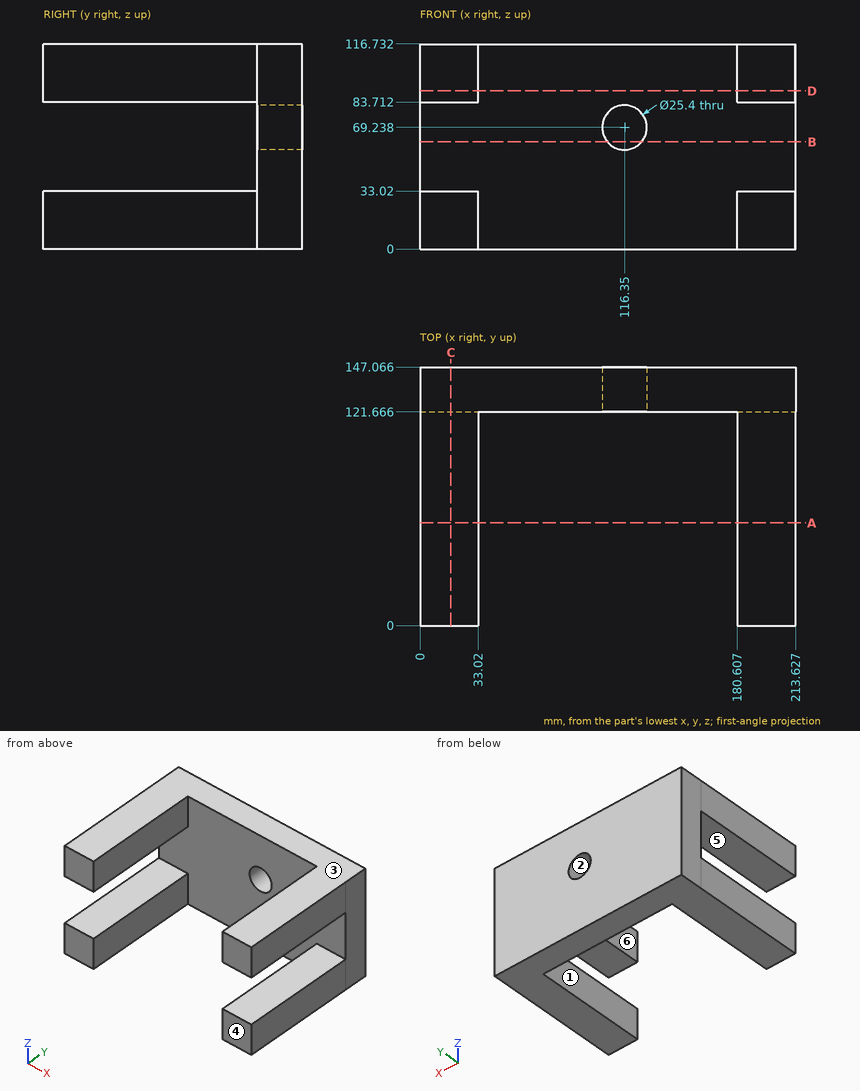
Can you work these out from the drawing? Everything is in mm from the part's minimum corner. A direction names the side the tool comes from. Round coordinates to 2 decimals unless told otherwise and drop trailing zeros. Order: outer loops, then holes, each group sorted by start corner. A loop starts at its lowest first (then second) coordinate and runs counter-clockwise, first axis right, second up. Notation, with made-up numbers: (63, 6.5) -> (114, 6.5) arc R26 ccw to (114, 40.5) -> close; hole circle Ø10 at (-36, 68). An arc over 180 degrees is marked (long way). Return JSON: item names as keys, results as strings. Group by question number.
1. I need wall thicknesses on line 1 (X direction, y = 59, z = 10.5); line 2 (Z direction, x = 205, y = 98); line 3 (Y direction, x = 205.5, z = 36). Which ranges of each line are inside material? Lowest first, please. Write a range as [from, to].
2. We'd pull the mould along Z, two halves only. Please class the marked faces 1, 2 and 3: released by +Z, released by -Z, zero draft, split by the parting line, or undercut.
3. If we section it at A-A, the plane y = 58.5: Write out the boundary of the cut face in (x, z), then the cut area to 3 significant figures.
4. If we section it at D-D, the plane z = 90: Write out the boundary of the cut face in (x, y), then the cut area to 3 significant figures.
5. Will this pin go through, and if not, where does the flat tip stop? pin 1 (6 mm diameter, centred on x = 35.5, z = 11.5, fed in from -Y).
6. If we section it at C-C, the plane x = 17.5: Write out the boundary of the cut face in (y, z), then the cut area to 3 significant figures.
7. If we section it at B-B, the plane z = 61: Write out the boundary of the cut face in (x, y) (1 decimal).
8. Which directions (+Z, -Z, +X, -X, +Y, -Y) give clear straight access to the entire face, cutting with the end or side of a thin tool? Please do the marked faces 4, 5 and 6.
Output values:
{
 "1": {"line 1": "[0, 33.02], [180.61, 213.63]", "line 2": "[0, 33.02], [83.71, 116.73]", "line 3": "[121.67, 147.07]"},
 "2": {"face 1": "zero draft", "face 2": "undercut", "face 3": "released by +Z"},
 "3": {"outline": "(0, 0) -> (33.02, 0) -> (33.02, 33.02) -> (0, 33.02) -> close; (0, 83.71) -> (33.02, 83.71) -> (33.02, 116.73) -> (0, 116.73) -> close; (180.61, 0) -> (213.63, 0) -> (213.63, 33.02) -> (180.61, 33.02) -> close; (180.61, 83.71) -> (213.63, 83.71) -> (213.63, 116.73) -> (180.61, 116.73) -> close", "area": "4,360 mm²"},
 "4": {"outline": "(0, 0) -> (33.02, 0) -> (33.02, 121.67) -> (180.61, 121.67) -> (180.61, 0) -> (213.63, 0) -> (213.63, 147.07) -> (0, 147.07) -> close", "area": "13,500 mm²"},
 "5": {"pin 1": "y = 0"},
 "6": {"outline": "(0, 0) -> (147.07, 0) -> (147.07, 116.73) -> (0, 116.73) -> (0, 83.71) -> (121.67, 83.71) -> (121.67, 33.02) -> (0, 33.02) -> close", "area": "11,000 mm²"},
 "7": {"outline": "(0, 121.7) -> (106.7, 121.7) -> (106.7, 147.1) -> (0, 147.1) -> close; (126, 121.7) -> (213.6, 121.7) -> (213.6, 147.1) -> (126, 147.1) -> close"},
 "8": {"face 4": "+Z, -Z, +X, -X, -Y", "face 5": "+X, -X, -Y", "face 6": "+Z, -Z, -Y"}
}
